Answer from the drawing. Dimensions are ordinates in mm from the lowest x, y and z of the part. Give positions to 0.01 mm unless a question says otherwise; leave off trailing zeros. Write each loop counter-clockwise with the first axis right and the second up, starting at its lowest first coordinate (ties: lowest second). Pieces come first, ordered by that corner, then holes. Notation, with made-up numbers: (-4.5, -25) -> (30.5, -25) arc R24 ccw to (30.5, -11) -> close; hole circle Ø10 at (23.25, 2). An arc over 180 degrees is marked (long way). Use a Markdown table: item, result. Add a question column.
Q1. Section C-C, the plane x = 62 is taken. Give the vertices of the cut face in (y, z), plus the area to 3 significant figures.
Q2. Section B-B, the plane z = 10 is taken. Give the vertices of the cut face in (x, y), plus the area to 3 significant figures.
Q3. Section A-A, the plane x = 10 is taken. Give the vertices of the cut face in (y, z), plus the area to 3 significant figures.
Q4. This flat-tipped pin is pushed along its axis until it touches: pin 1 Ø3 at (x, z) = (90, 10) entering from +Y. Where does it stop, or does it pass through?
Q5. Consider line 1 (X direction, y = 2.2, z = 10.25); line 2 (Z direction, x = 10, y = 2.95); line 3 (X direction, y = 0.9, z = 10.5). Determine where each line is inside the solid, lowest interval first.
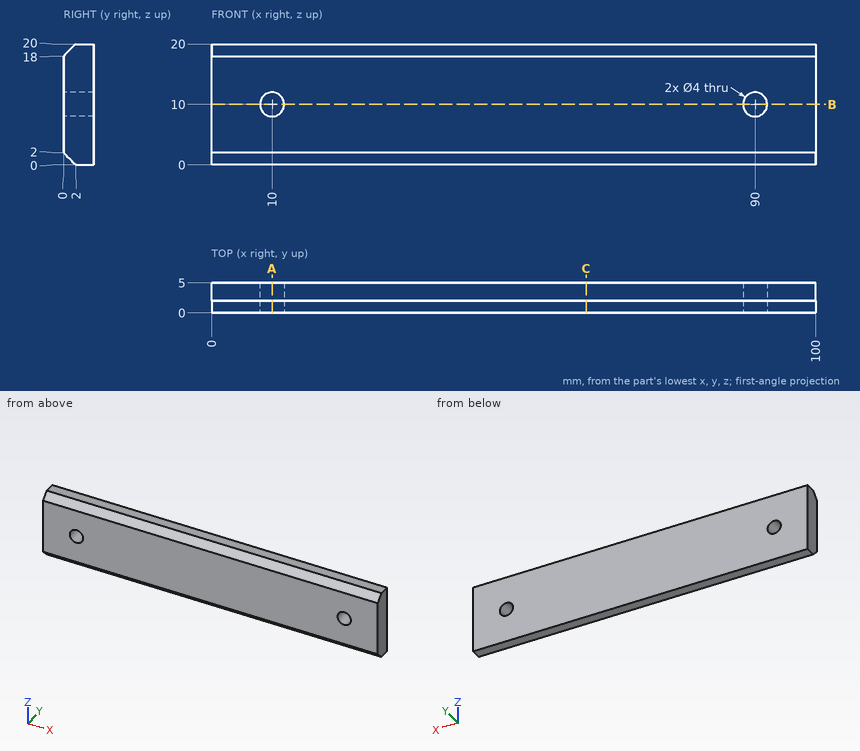
Result set:
| question | item | result |
|---|---|---|
| 1 | outline | (0, 2) -> (2, 0) -> (5, 0) -> (5, 20) -> (2, 20) -> (0, 18) -> close |
| 1 | area | 96.0 mm2 |
| 2 | outline | (0, 0) -> (8, 0) -> (8, 5) -> (0, 5) -> close; (12, 0) -> (88, 0) -> (88, 5) -> (12, 5) -> close; (92, 0) -> (100, 0) -> (100, 5) -> (92, 5) -> close |
| 2 | area | 460 mm2 |
| 3 | outline | (0, 2) -> (2, 0) -> (5, 0) -> (5, 8) -> (0, 8) -> close; (0, 12) -> (5, 12) -> (5, 20) -> (2, 20) -> (0, 18) -> close |
| 3 | area | 76.0 mm2 |
| 4 | pin 1 | passes through |
| 5 | line 1 | x = 0 to 8.02, 11.98 to 88.02, 91.98 to 100 |
| 5 | line 2 | z = 0 to 8, 12 to 20 |
| 5 | line 3 | x = 0 to 8.06, 11.94 to 88.06, 91.94 to 100 |
